Autodesk Inventor part; units mm, degrees
ref_plane "YZ Plane" through (0, 0, 0) normal (1, 0, 0) x (0, 1, 0)
ref_plane "XZ Plane" through (0, 0, 0) normal (0, 1, 0) x (-1, 0, 0)
ref_plane "XY Plane" through (0, 0, 0) normal (0, 0, 1) x (1, 0, 0)
sketch "Sketch1" plane through (0, 0, 0) normal (1, 0, 0) x (0, 1, 0)
  line L0 (-16.0539, 66.6862) -> (18.9461, 66.6862)
  line L1 (23.9461, 61.6862) -> (23.9461, -29.3138)
  line L2 (-21.0539, -29.3138) -> (-21.0539, 61.6862)
  circle A0 centre (-6.3039, -8.3138) radius 1.75
  circle A1 centre (1.4461, -16.0638) radius 1.75
  circle A2 centre (9.1961, -8.3138) radius 1.75
  circle A3 centre (1.4461, -0.5638) radius 1.75
  circle A4 centre (1.4461, 16.6862) radius 4
  line L3 (-21.0539, -29.3138) -> (23.9461, -29.3138)
  circle A5 centre (17.1961, 16.6862) radius 2.8
  circle A6 centre (1.4461, -8.3138) radius 4
  circle A7 centre (-14.3039, 16.6862) radius 2.8
  arc A8 (-16.0539, 66.6862) -> (-21.0539, 61.6862) centre (-16.0539, 61.6862) ccw
  arc A9 (23.9461, 61.6862) -> (18.9461, 66.6862) centre (18.9461, 61.6862) ccw
  circle A10 centre (-5.5539, 56.6862) radius 1.75
  circle A11 centre (8.4461, 56.6862) radius 1.75
  point P0 (0, 0)
  point P1 (-21.0539, 66.6862)
  point P2 (23.9461, 66.6862)
  dimension "d4" = 360
  dimension "d7" = 8
  dimension "d15" = 8
  dimension "d16" = 5.6
  dimension "d20" = 5.6
  dimension "d21" = 31.5
  dimension "d22" = 15.75
  dimension "d23" = 25
  dimension "d25" = 5
  dimension "d26" = 45
  dimension "d28" = 22.5
  dimension "d29" = 14
  dimension "d30" = 15.5
  dimension "d31" = 3.5
  dimension "d32" = 3.5
  dimension "d33" = 91
  dimension "d34" = 10
extrude "Extrusion1" add sketch "Sketch1" along normal blind 6.35 contours L0 A9 L1 L3 L2 A8 | A0 | A1 | A2 | A3
equation "\"d28\" = 0.5 * d26"
properties part number "carriage"
Source: CAD feature listing. Evaluate the final solid. Frame: model axes, mm. Round coordinates to 2 decimals unless told otherwise and drop trailing zeros. Order: outer loops, then holes, each group sorted by start corner. A loop starts at its lowest first (then second) coordinate and runs counter-clockwise, first axis right, second up. Notation, with made-up numbers: (62.5, 37.5) - (93.5, 37.5) arc R22 cw to (93.5, 64.5) - close; hole circle Ø8 at (-32, 54). An arc over 180 degrees is marked (long way). Use a Markdown table: item, result. Add a question column.
1. Section query D-D (z = -10). Return the cut outline in (x, y).
2. Section query A-A (y = 4). Return the cut outline in (x, z).
3. First-contact query: pin 1 (5 mm diameter, centred on y = 1.45, z = 16.69, fed in from +X). Flat tip, straight axial feed; report the tip coordinate or a pass-through.
4. Section query B-B (y = 9). Return the cut outline in (x, z).
5. Mould query, pull axis Z, two halves, no side actions, for faces 1 (the flat face through (3, 1, 66.686)), 2 (the flat face through (3, 23.946, 17)), 3 (the cylindrical face through (3.13, 0.93, -12.28)). Classes: +Z half, -Z half, draft (parallel to the pull), parting line (faces both ways), or undercut.
6. Section query C-C (x = 2.5). Return the cut outline in (y, z), then the cut area to 3 significant figures.
7. Line query: probe 1 along Z at (x, y) = (3.5, 2); probe 2 along Y at (x, z) = (6, 56); probe 3 along Z at (x, y) = (3.25, -15). Output: solid intervals per line, ascending.
Derived:
| question | item | result |
|---|---|---|
| 1 | outline | (0, -21.05) - (6.35, -21.05) - (6.35, -2.18) - (0, -2.18) - close; (0, 5.07) - (6.35, 5.07) - (6.35, 23.95) - (0, 23.95) - close |
| 2 | outline | (0, -29.31) - (6.35, -29.31) - (6.35, -11.39) - (0, -11.39) - close; (0, -5.24) - (6.35, -5.24) - (6.35, 13.61) - (0, 13.61) - close; (0, 19.76) - (6.35, 19.76) - (6.35, 66.69) - (0, 66.69) - close |
| 3 | pin 1 | through |
| 4 | outline | (0, -29.31) - (6.35, -29.31) - (6.35, 55.03) - (0, 55.03) - close; (0, 58.35) - (6.35, 58.35) - (6.35, 66.69) - (0, 66.69) - close |
| 5 | face 1 | +Z half |
| 5 | face 2 | draft |
| 5 | face 3 | undercut |
| 6 | outline | (-21.05, -29.31) - (23.95, -29.31) - (23.95, 61.69) arc R5 ccw to (18.95, 66.69) - (-16.05, 66.69) arc R5 ccw to (-21.05, 61.69) - close; hole circle Ø5.6 at (-14.3, 16.69); hole circle Ø3.5 at (-5.55, 56.69); hole circle Ø8 at (1.45, -8.31); hole circle Ø8 at (1.45, 16.69); hole circle Ø3.5 at (8.45, 56.69); hole circle Ø5.6 at (17.2, 16.69) |
| 6 | area | 4,140 mm2 |
| 7 | probe 1 | -29.31 to -12.28, -4.35 to 12.72, 20.65 to 66.69 |
| 7 | probe 2 | -21.05 to -7.16, -3.94 to 6.84, 10.06 to 23.95 |
| 7 | probe 3 | -29.31 to 13.97, 19.4 to 66.69 |
